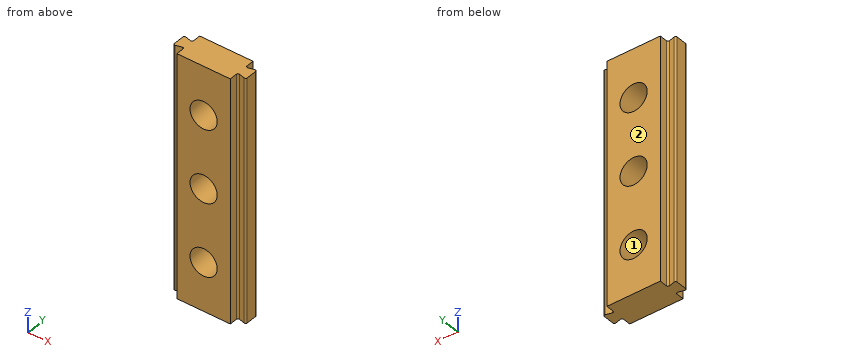
```python
from build123d import *

# Parameters (mm, degrees)
SALIENTE_EXTRUIR1_DEPTH      = 3
SALIENTE_EXTRUIR1_DEPTH_BACK = 3
CROQUIS1_W                   = 15
CROQUIS1_H                   = 50
TALADRO1_D                   = 5.6
CORTAR_EXTRUIR2_DEPTH        = 27.272609311
REDONDEO1_R                  = 0.3
REDONDEO1_OF_SIMETR_A1_R     = 0.3
SIMETR_A2_START              = -25
SIMETR_A2_DEPTH              = 50


# Read off the part's stored shape, not the designer's step: Simetría2
with BuildPart() as part:
    # Croquis1 → Saliente-Extruir1 (new, two sides: drawn at the far end of the back side and taken through both)
    with BuildSketch(Plane(origin=(0, 0, 0), x_dir=(1, 0, 0), z_dir=(0, 1, 0)).offset(-SALIENTE_EXTRUIR1_DEPTH_BACK)):
        Rectangle(CROQUIS1_W, CROQUIS1_H)
    extrude(amount=SALIENTE_EXTRUIR1_DEPTH + SALIENTE_EXTRUIR1_DEPTH_BACK)

    # Taladro1 (through all)
    with Locations(Plane(origin=(0, 3, 0), x_dir=(1, 0, 0), z_dir=(0, 1, 0))):
        with Locations((0, 15), (0, -15), (0, 0)):
            Hole(TALADRO1_D / 2)

    # Croquis5 → Cortar-Extruir2 (cut, symmetric)
    with BuildSketch(Plane.XY):
        Polygon((5.5, -3), (5.5, -1), (7.5, -1.5), (7.5, -3), align=None)
    cortar_extruir2 = extrude(amount=CORTAR_EXTRUIR2_DEPTH, both=True, mode=Mode.SUBTRACT)

    # Redondeo1
    redondeo1_edges = [part.edges().sort_by_distance(p)[0] for p in [
        (5.5, -1, 0),
        (7.5, -1.5, 0),
    ]]
    fillet(redondeo1_edges, radius=REDONDEO1_R)

    # Simetría1: Cortar-Extruir2 across plane
    add(cortar_extruir2.mirror(Plane.ZX), mode=Mode.SUBTRACT)

    # Redondeo1 of Simetría1
    redondeo1_of_simetr_a1_edges = [part.edges().sort_by_distance(p)[0] for p in [
        (5.5, 1, 0),
        (7.5, 1.5, 0),
    ]]
    fillet(redondeo1_of_simetr_a1_edges, radius=REDONDEO1_OF_SIMETR_A1_R)

    # Simetría2 outline → Simetría2 (cut)
    with BuildSketch(Plane.XY.offset(SIMETR_A2_START)):
        with BuildLine():
            Line((-7.5, -3), (-5.5, -3))
            Line((-5.5, -3), (-5.5, -1.384232922))
            ThreePointArc((-5.5, -1.384232922), (-5.615376338, -1.147771291), (-5.872760688, -1.093190172))
            Line((-5.872760688, -1.093190172), (-7.127239312, -1.406809828))
            ThreePointArc((-7.127239312, -1.406809828), (-7.384623662, -1.352228709), (-7.5, -1.115767078))
            Line((-7.5, -1.115767078), (-7.5, -3))
        make_face()
        with BuildLine():
            Line((-7.5, 3), (-7.5, 1.115767078))
            ThreePointArc((-7.5, 1.115767078), (-7.384623662, 1.352228709), (-7.127239312, 1.406809828))
            Line((-7.127239312, 1.406809828), (-5.872760688, 1.093190172))
            ThreePointArc((-5.872760688, 1.093190172), (-5.615376338, 1.147771291), (-5.5, 1.384232922))
            Line((-5.5, 1.384232922), (-5.5, 3))
            Line((-5.5, 3), (-7.5, 3))
        make_face()
    extrude(amount=SIMETR_A2_DEPTH, mode=Mode.SUBTRACT)


solid = part.part
```
The model under review builds one solid part; all positions refer to its coordinate system, in mm. Face numbers are marked on the shaded views. Coordinates: 2 decimals unless noted, no trailing zeros. Write each loop counter-clockwise with the first axis right and the second up, starting at its lowest first coordinate (ties: lowest second). Pieces come first, ordered by that corner, then holes. Notation, with made-up numbers: (28.25, -25) -> (74.25, -25) arc R32 ccw to (74.25, 11) -> close; hole circle Ø6 at (8.5, 13). An arc over 180 degrees is marked (long way). One line per item, written item: value. Start each with the question number.
Q1. Add section C-C, the plane y = 0.05. Give the boundary of the cut face in (x, z), then the cut area to 3 significant figures.
Q2. The part is to be moulded in two halves that separate along X. For the marked faces 1 and 2, say which applies: +X half, -X half, draft (parallel to the pull), parting line (faces both ways), or undercut.
Q3. Add section A-A, the plane z = 0. Give the boundary of the cut face in (x, y), then the cut area to 3 significant figures.
Q4. To check wall thickness, follow probe 1 along Z at (x, y) = (0, -0.9); probe 2 along X at (y, z) = (-1.05, -15); probe 3 along Z at (x, y) = (2.5, -0.8). State the ranges of each line that lie inside material, in increasing order.
Q5. Clearance check with flat-ended pins moving along their axes: P1, Ø5, axis at x = 0, z = -15, coming from the -Y side; P2, Ø1.8, axis at y = 2, z = 8, coming from the -X side; P3, Ø0.8, axis at y = -2, z = 0.5, coming from the -X side. State where each tip first meets the part, or that it passes through.
Q6. Add section B-B, the plane x = 0. Give the boundary of the cut face in (y, z), then the cut area to 3 significant figures.
Q7. Add section D-D, the plane z = -14. Give the boundary of the cut face in (x, y).
Response:
1. outline: (-7.5, -25) -> (7.5, -25) -> (7.5, 25) -> (-7.5, 25) -> close; hole circle Ø5.6 at (0, -15); hole circle Ø5.6 at (0, 0); hole circle Ø5.6 at (0, 15)
1. area: 676 mm²
2. face 1: undercut
2. face 2: draft
3. outline: (-7.5, -1.12) arc R0.3 ccw to (-7.13, -1.41) -> (-5.87, -1.09) arc R0.3 cw to (-5.5, -1.38) -> (-5.5, -3) -> (-2.8, -3) -> (-2.8, 3) -> (-5.5, 3) -> (-5.5, 1.38) arc R0.3 cw to (-5.87, 1.09) -> (-7.13, 1.41) arc R0.3 ccw to (-7.5, 1.12) -> close; (2.8, -3) -> (5.5, -3) -> (5.5, -1.38) arc R0.3 cw to (5.87, -1.09) -> (7.13, -1.41) arc R0.3 ccw to (7.5, -1.12) -> (7.5, 1.12) arc R0.3 ccw to (7.13, 1.41) -> (5.87, 1.09) arc R0.3 cw to (5.5, 1.38) -> (5.5, 3) -> (2.8, 3) -> close
3. area: 42.4 mm²
4. probe 1: -25 to -17.8, -12.2 to -2.8, 2.8 to 12.2, 17.8 to 25
4. probe 2: -7.5 to -2.8, 2.8 to 7.5
4. probe 3: -25 to -16.26, -13.74 to -1.26, 1.26 to 13.74, 16.26 to 25
5. P1: through
5. P2: x = -7.5
5. P3: x = -5.5
6. outline: (-3, -25) -> (3, -25) -> (3, -17.8) -> (-3, -17.8) -> close; (-3, -12.2) -> (3, -12.2) -> (3, -2.8) -> (-3, -2.8) -> close; (-3, 2.8) -> (3, 2.8) -> (3, 12.2) -> (-3, 12.2) -> close; (-3, 17.8) -> (3, 17.8) -> (3, 25) -> (-3, 25) -> close
6. area: 199 mm²
7. outline: (-7.5, -1.12) arc R0.3 ccw to (-7.13, -1.41) -> (-5.87, -1.09) arc R0.3 cw to (-5.5, -1.38) -> (-5.5, -3) -> (-2.62, -3) -> (-2.62, 3) -> (-5.5, 3) -> (-5.5, 1.38) arc R0.3 cw to (-5.87, 1.09) -> (-7.13, 1.41) arc R0.3 ccw to (-7.5, 1.12) -> close; (2.62, -3) -> (5.5, -3) -> (5.5, -1.38) arc R0.3 cw to (5.87, -1.09) -> (7.13, -1.41) arc R0.3 ccw to (7.5, -1.12) -> (7.5, 1.12) arc R0.3 ccw to (7.13, 1.41) -> (5.87, 1.09) arc R0.3 cw to (5.5, 1.38) -> (5.5, 3) -> (2.62, 3) -> close
